```python
from build123d import *

# Parameters (mm, degrees)
SKETCH1_W           = 35
SKETCH1_H           = 7
BOSS_EXTRUDE1_DEPTH = 5
SKETCH2_R           = 1.45
SKETCH2_R_2         = 1.6
CUT_EXTRUDE1_DEPTH  = 37.041642582
FILLET1_R           = 3


with BuildPart() as part:
    # Sketch1 → Boss-Extrude1 (new body)
    with BuildSketch(Plane(origin=(0, 0, 0), x_dir=(0, 0, -1), z_dir=(1, 0, 0))):
        with Locations((17.5, -3.5)):
            Rectangle(SKETCH1_W, SKETCH1_H)
    extrude(amount=BOSS_EXTRUDE1_DEPTH)

    # Sketch2 → Cut-Extrude1 (cut, through all)
    with BuildSketch(Plane(origin=(5, 0, 0), x_dir=(0, 0, -1), z_dir=(1, 0, 0))):
        with Locations((4, -3.5)):
            Circle(SKETCH2_R)
        with Locations((12.2, -3.5)):
            Circle(SKETCH2_R)
        with Locations((31, -3.5)):
            Circle(SKETCH2_R_2)
    extrude(amount=-CUT_EXTRUDE1_DEPTH, mode=Mode.SUBTRACT)

    # Fillet1
    fillet1_edges = [part.edges().sort_by_distance(p)[0] for p in [
        (2.5, 0, 0),
        (2.5, 0, -35),
        (2.5, -7, -35),
        (2.5, -7, 0),
    ]]
    fillet(fillet1_edges, radius=FILLET1_R)


solid = part.part
```
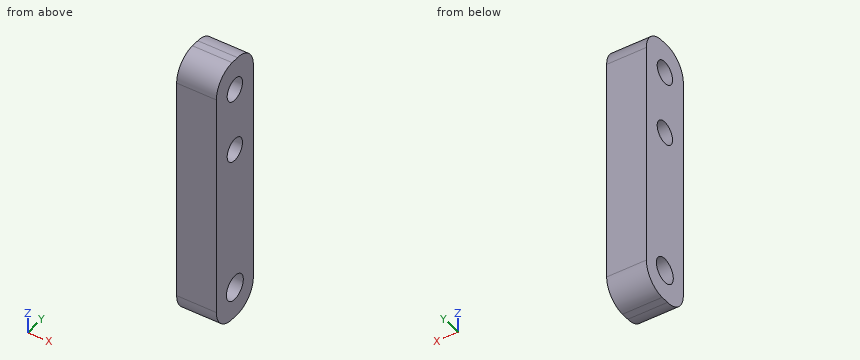
Could you check a few things on this model? Use its own coordinates, in mm. Round coordinates to 2 decimals unless told otherwise and drop trailing zeros. Loops run counter-clockwise (first coordinate to the right, second up) from the corner with the lowest first, then second, coordinate; pieces in that order, holes last. Notation, with made-up numbers: (14.25, -16.75) - (33.25, -16.75) arc R19 cw to (33.25, -6.75) - close; hole circle Ø6 at (20, 27.25). An arc over 180 degrees is marked (long way). Answer in a Markdown table with one row per item. Add a question column.
(1) I need wall thicknesses on line 1 along Y through (x, z) = (2.8, -31); line 2 along Y through (x, z) = (1.7, -4); line 3 along Z through (x, y) = (2, -3.25). Which ranges of each line are inside material? Lowest first, please.
(2) If we section it at D-D (y = -6.25): Please give me the cut outline in (x, z), plus the area to 3 significant figures.
(3) If we section it at A-A (z = -31): Please give me the cut outline in (x, y).
(4) If we section it at C-C (z = -12.2): Please give me the cut outline in (x, y), plus the area to 3 significant figures.
(5) I'm going to push a flat-ended pin straight in: pin 1 (1 mm diameter, centred on y = -5, z = -5.5, fed in from -X). Where does the tip first touch, or does it pass through?
(6) If we section it at B-B (x = 3.55): Please give me the cut outline in (y, z).
Model answer:
| question | item | result |
|---|---|---|
| 1 | line 1 | y = -7 to -5.1, -1.9 to 0 |
| 1 | line 2 | y = -7 to -4.95, -2.05 to 0 |
| 1 | line 3 | z = -35 to -32.58, -29.42 to -13.63, -10.77 to -5.43, -2.57 to 0 |
| 2 | outline | (0, -33.98) - (5, -33.98) - (5, -1.02) - (0, -1.02) - close |
| 2 | area | 165 mm² |
| 3 | outline | (0, -7) - (5, -7) - (5, -5.1) - (0, -5.1) - close; (0, -1.9) - (5, -1.9) - (5, 0) - (0, 0) - close |
| 4 | outline | (0, -7) - (5, -7) - (5, -4.95) - (0, -4.95) - close; (0, -2.05) - (5, -2.05) - (5, 0) - (0, 0) - close |
| 4 | area | 20.5 mm² |
| 5 | pin 1 | stops at x = 0 |
| 6 | outline | (-7, -32) arc R3 ccw to (-4, -35) - (-3, -35) arc R3 ccw to (0, -32) - (0, -3) arc R3 ccw to (-3, 0) - (-4, 0) arc R3 ccw to (-7, -3) - close; hole circle Ø3.2 at (-3.5, -31); hole circle Ø2.9 at (-3.5, -12.2); hole circle Ø2.9 at (-3.5, -4) |
